Geometry check sheet. Reference: the model listing, model coordinates, mm. A direction names the side the tool comes from. Give positions to 0.01 mm unless a question says otherwise; leave off trailing zeros. Write each loop counter-clockwise with the first axis right and the second up, starting at its lowest first coordinate (ties: lowest second). Pieces come first, ordered by that corner, then holes. Notation, with made-up numbers: (84.5, 77.5) - (117.5, 77.5) arc R36 cw to (117.5, 116.5) - close; hole circle Ø8 at (-4, 77.5). An arc over 180 degrees is marked (long way). Write item = value, one per line. Start each with the question number.
(1) Draft check along Y on faces 1 (the cylindrical face through (7.349, 26.925, 7.755)), 2 (the cylindrical face through (-5.636, 13.837, 8.291)), 3 (the flat face through (-4.65, 17, 22)). Enter one of: pulls with the +Y half, pulls with the -Y half, needs draft (parallel to the pull), parting line crosses it, or undercut.
(2) Section check C-C, the plane x = 0.5. Enter the section's corners in (y, z).
(3) Section check B-B, the plane x = -2.5. Enter the section's corners in (y, z), plus the area to 3 significant figures.
(4) Depth check by flat-ended pin: pin 1 Ø12 at (y, z) = (10, 10.5) entering from +X; pin 2 Ø2 at (x, z) = (0, 19.5) entering from +Y; pin 3 Ø2 at (x, z) = (5.5, 36.5) entering from -Y; pin 4 Ø6 at (y, z) = (8.5, 17.5) entering from +X. Enter the tip coordinate at first touch or a pass-through.
(5) Section check A-A, the plane x = 5.5. Enter the section's corners in (y, z), plus the area to 3 significant figures.
(6) Access from +Z, -Z, +X, -X, +Y, -Y to the whole of each face (thin tool, end or side, straight path). Record for faces 4 (the cylindrical face through (-7.4, 11.6, 16.7)), 5 (the flat face through (-5.636, 11.286, 16.566)), 6 (the flat face through (4.65, 17, 22)), 7 (the flat face through (0.1, 18.8, 21.7)), 8 (the cylindrical face through (-3.65, 25.79, 4.33)).
(7) Thickness scan on L1, parallel to X at y = 23.5, z = 13.5; L2, parallel to Y at x = 3.5, z = 17; L3, parallel to Z at x = -4, y = 20.5. Record the ranges inside material, lowest first.
```python
from build123d import *

# Parameters (mm, degrees)
PAD004_DEPTH            = 7.65
POCKET003_DEPTH         = 4.65
POCKET004_DEPTH         = 2
FILLET007_R             = 1
FILLET008_R             = 1
BODY003_PLACEMENT_ANGLE = 289


with BuildPart() as part:
    # Sketch009 → Pad004 (new body, symmetric)
    with BuildSketch(Plane.YZ):
        with BuildLine():
            ThreePointArc((-2.8284271247, -1), (-0.1735950846, -2.9949732464), (2.6939497909, -1.3200888318))
            Line((2.6939497909, -1.3200888318), (7.8, 9.1))
            Line((7.8, 9.1), (-3.7, 14.7352281014))
            ThreePointArc((-3.7, 14.7352281014), (-4.158961759, 14.9368094594), (-4.6331484619, 15.0993760945))
            Line((-4.6331484619, 15.0993760945), (-28.6904310189, 22.2388309237))
            ThreePointArc((-28.6904310189, 22.2388309237), (-33.6993372116, 18.5718979166), (-28.8290152057, 14.7228067922))
            Line((-27.5290152057, 11.9228067922), (-28.8290152057, 14.7228067922))
            ThreePointArc((-27.5290152057, 11.9228067922), (-29.4749197629, 5.5883007232), (-29.9826934773, -1.0188679245))
            ThreePointArc((-29.9826934773, -1.0188679245), (-27.4803397166, -4.255402597), (-23.6176804166, -2.9075175272))
            Line((-23.6176804166, -2.9075175272), (-22.4775697078, -1.2792706909))
            ThreePointArc((-20.0201135749, 0), (-21.4053594146, -0.3389675005), (-22.4775697078, -1.2792706909))
            Line((-4.2426406871, 0), (-20.0201135749, 0))
            ThreePointArc((-2.8284271247, -1), (-3.3766152833, -0.2752551286), (-4.2426406871, 0))
        make_face()
    extrude(amount=PAD004_DEPTH, both=True)

    # Sketch010 → Pocket003 (cut, symmetric)
    with BuildSketch(Plane.YZ):
        with BuildLine():
            Line((6.9199407788, 7.3040334727), (-5.8060355253, 13.5400142802))
            ThreePointArc((-5.8060355253, 13.5400142802), (-11.1364622888, 12.5033421393), (-11.5881769744, 7.0918642957))
            Line((-11.5881769744, 7.0918642957), (-7.7326639328, 1.0024084327))
            Line((-9, 0.2), (-7.7326639328, 1.0024084327))
            Line((-9, 0.2), (-20, 17.5735670895))
            Line((-24.6418524264, 18.9511248267), (-20, 17.5735670895))
            ThreePointArc((-24.6418524264, 18.9511248267), (-25.4821110434, 18.8237971917), (-25.9209782539, 18.0960318164))
            ThreePointArc((-28.8290152057, 14.7228067922), (-26.8461376765, 15.9534931036), (-25.9209782539, 18.0960318164))
            Line((-28.8290152057, 14.7228067922), (-34.6400816793, 13.2289840317))
            Line((-34.6400816793, 13.2289840317), (-31.0800592212, -4.6959665273))
            Line((-31.0800592212, -4.6959665273), (6.9199407788, -4.6959665273))
            Line((6.9199407788, -4.6959665273), (6.9199407788, 7.3040334727))
        make_face()
    extrude(amount=POCKET003_DEPTH, both=True, mode=Mode.SUBTRACT)

    # Sketch011 (on Face6 of Pocket003) → Pocket004 (cut)
    with BuildSketch(Plane(origin=(0, 5.1060502091, 10.4200888318), x_dir=(0, -0.8979832636, 0.4400296106), z_dir=(0, 0.4400296106, 0.8979832636))):
        with BuildLine():
            Line((-3, 4.65), (-2, 4.65))
            ThreePointArc((1.5, 1.15), (0.4748737342, 3.6248737342), (-2, 4.65))
            Line((1.5, 1.15), (1.5, -1.15))
            ThreePointArc((-2, -4.65), (0.4748737342, -3.6248737342), (1.5, -1.15))
            Line((-2, -4.65), (-3, -4.65))
            Line((-3, -4.65), (-3, 4.65))
        make_face()
    extrude(amount=-POCKET004_DEPTH, mode=Mode.SUBTRACT)

    # Fillet007
    fillet007_edges = [part.edges().sort_by_distance(p)[0] for p in [
        (-6.15, 7.8, 9.1),
        (6.15, 7.8, 9.1),
    ]]
    fillet(fillet007_edges, radius=FILLET007_R)

    # Fillet008
    fillet008_edges = [part.edges().sort_by_distance(p)[0] for p in [
        (7.65, -16.66179, 18.669104),
        (-7.65, -16.66179, 18.669104),
        (-7.65, -28.179015, 13.322807),
        (7.65, -28.179015, 13.322807),
    ]]
    fillet(fillet008_edges, radius=FILLET008_R)


with BuildPart() as part_1:
    # Body003 placement: moved
    add(part.part.moved(Location((0, 15.2, 5.2))).rotate(Axis((0, 15.2, 5.2), (1, 0, 0)), BODY003_PLACEMENT_ANGLE))


solid = part_1.part
```
Model answer:
q1.face_1 = pulls with the +Y half
q1.face_2 = pulls with the -Y half
q1.face_3 = undercut
q2.outline = (12.46, 13.77) - (13.63, 12.84) - (18.13, 18.47) arc R4.5 cw to (26.11, 15.1) - (24.92, 5.5) - (26.9, 5.25) - (27.93, 13.5) arc R6 ccw to (27.97, 14.5) - (26.89, 39.57) arc R3.9 ccw (long way) to (23.87, 35.6) arc R1 cw to (25.1, 34.67) - (25.3, 29.83) - close
q3.outline = (12.46, 13.77) - (13.63, 12.84) - (18.13, 18.47) arc R4.5 cw to (26.11, 15.1) - (24.88, 5.23) - (26.87, 4.98) - (27.93, 13.5) arc R6 ccw to (27.97, 14.5) - (26.89, 39.57) arc R3.9 ccw (long way) to (23.87, 35.6) arc R1 cw to (25.1, 34.67) - (25.3, 29.83) - close
q3.area = 168 mm²
q4.pin_1 = 7.65
q4.pin_2 = 27.8
q4.pin_3 = 17.91
q4.pin_4 = 7.59
q5.outline = (4.48, 33.22) arc R3.5 ccw to (4.76, 26.58) - (6.67, 26.04) arc R3 cw to (8.68, 24.13) - (13.82, 9.21) arc R1.5 cw to (13.33, 7.55) arc R3 ccw to (14.83, 2.22) - (25.35, 0.91) arc R1 ccw to (26.47, 1.78) - (27.93, 13.5) arc R6 ccw to (27.97, 14.5) - (26.89, 39.57) arc R3.9 ccw (long way) to (19.73, 37.25) - (17.51, 35.11) arc R30 ccw to start
q5.area = 659 mm²
q6.face_4 = -X, -Y
q6.face_5 = +X, -X, -Y
q6.face_6 = none
q6.face_7 = -Y
q6.face_8 = -Z, -Y
q7.L1 = -7.65 to -4.65, 4.65 to 7.65
q7.L2 = 15.04 to 16.96, 25.94 to 27.86
q7.L3 = 20.01 to 23.83, 36.4 to 42.4
